```python
from build123d import *

# Parameters (mm, degrees)
F0_W     = 38.1
F0_H     = 19.05
F1_DEPTH = 3.175
F2_R     = 2.4828109925
F3_DEPTH = 3.176
F4_R     = 2.4828109925
F4_R_2   = 3.3973385268
F4_R_3   = 3.0356553695
F5_DEPTH = 0.254


with BuildPart() as f1:
    # F0 (on Top) → F1 (new body)
    with BuildSketch(Plane.XY):
        with Locations((-19.05, 9.525)):
            Rectangle(F0_W, F0_H)
    extrude(amount=F1_DEPTH)

    # F2 (on face) → F3 (cut, through all)
    with BuildSketch(Plane.XY.offset(3.175)):
        with BuildLine():
            ThreePointArc((-38.1, 9.525), (-35.2368913149, 16.0874822179), (-28.718682006, 19.05))
            Line((-28.718682006, 19.05), (-38.1, 19.05))
            Line((-38.1, 19.05), (-38.1, 9.525))
        make_face()
        with BuildLine():
            ThreePointArc((-28.718682006, 0), (-35.2368913149, 2.9625177821), (-38.1, 9.525))
            Line((-38.1, 9.525), (-38.1, 0))
            Line((-38.1, 0), (-28.718682006, 0))
        make_face()
        with Locations((-33.7038896978, 9.525)):
            Circle(F2_R)
    extrude(amount=-F3_DEPTH, mode=Mode.SUBTRACT)

    # F4 (on face) → F5 (cut)
    with BuildSketch(Plane.XY.offset(3.175)):
        with BuildLine():
            ThreePointArc((-28.718682006, 19.05), (-35.2368913149, 16.0874822179), (-38.1, 9.525))
            ThreePointArc((-38.1, 9.525), (-35.2368913149, 2.9625177821), (-28.718682006, 0))
            Line((-28.718682006, 0), (0, 0))
            Line((0, 0), (0, 19.05))
            Line((0, 19.05), (-28.718682006, 19.05))
        make_face()
        with Locations((-33.7038896978, 9.525)):
            Circle(F4_R, mode=Mode.SUBTRACT)
        with BuildLine():
            Line((-11.204509369, 9.7731091082), (-16.2556674331, 9.7731091082))
            Line((-16.2556674331, 9.7731091082), (-16.6581426853, 9.7731091082))
            ThreePointArc((-16.6581426853, 9.7731091082), (-24.1825202508, 10.7437230347), (-16.6363575836, 11.5271629766))
            Line((-16.6363575836, 11.5271629766), (-16.3941457868, 11.5271629766))
            Line((-16.3941457868, 11.5271629766), (-11.2256935624, 11.5271629766))
            ThreePointArc((-11.2256935624, 11.5271629766), (-3.4717256344, 10.7436549328), (-11.204509369, 9.7731091082))
        make_face(mode=Mode.SUBTRACT)
        with Locations((-7.3930802755, 10.6962956488)):
            Circle(F4_R_2)
        with BuildLine():
            add(Edge.make_bspline(
                [(-8.4561556578, 10.4526774958), (-8.4344821955, 10.5131812711), (-8.6159052615, 10.7046403164), (-8.9098232628, 10.8195179836), (-9.3586544368, 10.7286119848), (-9.574745931, 10.1187053668), (-9.2805338199, 9.538167958), (-8.8082365512, 9.5804816092), (-8.4556586549, 9.7438202932), (-8.396860102, 9.9863555926), (-8.6330082393, 10.0702183652), (-8.6519010809, 9.7333768373), (-9.0449295596, 9.7024764863), (-9.3441221135, 9.9584577723), (-9.3874655572, 10.524078357), (-8.9264365843, 10.6826697258), (-8.6368050913, 10.6049347389), (-8.6279642917, 10.3475627852), (-8.4719713543, 10.4085262966), (-8.4561556578, 10.4526774958)],
                knots=[0, 0, 0, 0, 0.0532483387, 0.113267174, 0.1785434515, 0.2577982567, 0.3354252403, 0.4027712128, 0.4668510982, 0.5116274353, 0.551372775, 0.6028604887, 0.6613225245, 0.7248177023, 0.7963036394, 0.8635278137, 0.9167089689, 0.9611432841, 1, 1, 1, 1], degree=3))
        make_face(mode=Mode.SUBTRACT)
        Polygon((-8.2311294973, 9.6275797114), (-8.2311294973, 10.7419975102), (-8.0918269232, 10.7741439715), (-8.0918269232, 9.7133042291), (-7.5239026919, 9.7133042291), (-7.5239026919, 9.6275797114), align=None, mode=Mode.SUBTRACT)
        with BuildLine():
            Line((-6.3773384318, 10.7741439715), (-6.3773384318, 10.6962956488))
            Line((-6.3773384318, 10.6962956488), (-6.3773384318, 9.9276155233))
            add(Edge.make_bspline(
                [(-6.3773384318, 9.9276155233), (-6.4090453416, 9.8087981466), (-6.480236508, 9.5420188336), (-7.1453746708, 9.5677405448), (-7.258420068, 9.8154754172), (-7.3095913976, 9.9276155233)],
                knots=[0, 0, 0, 0, 0.3053274615, 0.6855482984, 1, 1, 1, 1], degree=3))
            Line((-7.3095913976, 9.9276155233), (-7.2881602682, 10.7955755666))
            Line((-7.2881602682, 10.7955755666), (-7.1702892892, 10.7926651697))
            Line((-7.1702892892, 10.7926651697), (-7.1702892892, 9.9276155233))
            add(Edge.make_bspline(
                [(-7.1702892892, 9.9276155233), (-7.1284542088, 9.8465309767), (-7.0391238846, 9.6733913827), (-6.6129016247, 9.6843481722), (-6.5685332878, 9.8526930406), (-6.5487870015, 9.9276155233)],
                knots=[0, 0, 0, 0, 0.3283233699, 0.7010679257, 1, 1, 1, 1], degree=3))
            Line((-6.5487870015, 9.9276155233), (-6.5487870015, 10.7741439715))
            Line((-6.5487870015, 10.7741439715), (-6.3773384318, 10.7741439715))
        make_face(mode=Mode.SUBTRACT)
        with BuildLine():
            Line((-6.1201648787, 9.6168639138), (-6.1201648787, 10.6962956488))
            Line((-6.1201648787, 10.6962956488), (-6.1201648787, 10.8170062304))
            Line((-6.1201648787, 10.8170062304), (-5.577086471, 10.8170062304))
            add(Edge.make_bspline(
                [(-5.577086471, 10.8170062304), (-5.4622781191, 10.7638193061), (-5.2295052196, 10.6559832962), (-5.3677642589, 10.2445065322), (-5.5472345904, 10.2120818848), (-5.1332134299, 10.1753596302), (-5.270141809, 9.5907558618), (-5.4344035608, 9.6095224454), (-5.498662591, 9.6168639138)],
                knots=[0, 0, 0, 0, 0.1903840672, 0.3860019817, 0.4771127011, 0.6375520727, 0.8582107397, 1, 1, 1, 1], degree=3))
            Line((-5.498662591, 9.6168639138), (-6.1201648787, 9.6168639138))
        make_face(mode=Mode.SUBTRACT)
        with BuildLine():
            add(Edge.make_bspline(
                [(-8.5740266368, 12.2743221), (-8.5401050741, 12.3224331664), (-8.6783215627, 12.6387800293), (-9.184796294, 12.6548329665), (-9.4800471983, 12.4360053833), (-9.4419740945, 12.0798316165), (-9.1295950241, 11.9793082685), (-8.831367579, 11.9123580888), (-8.6427968335, 11.8238895712), (-8.7645291474, 11.5344085895), (-9.1140370755, 11.5542180365), (-9.3260330715, 11.6778761827), (-9.2954318773, 11.9042158216), (-9.5962395192, 11.8814661597), (-9.3559672194, 11.4482164997), (-8.9967184633, 11.3933195663), (-8.5558015163, 11.4768320471), (-8.5479985096, 11.8327800081), (-8.6951902579, 12.1024272986), (-9.0540613983, 12.0793081599), (-9.2629319892, 12.2276324709), (-9.3267172394, 12.4649328799), (-8.8420264537, 12.5231376903), (-8.7560312169, 12.2648192132), (-8.5972865041, 12.2413325519), (-8.5740266368, 12.2743221)],
                knots=[0, 0, 0, 0, 0.0453790473, 0.1028040475, 0.1504811039, 0.1945666876, 0.2403101145, 0.2875747753, 0.3209496051, 0.3604616335, 0.4077131796, 0.4470225316, 0.4812881885, 0.5136946038, 0.5632768855, 0.6145773714, 0.6660910242, 0.7111117469, 0.7544039284, 0.8020681877, 0.8434151076, 0.8768269994, 0.927247352, 0.9688837855, 1, 1, 1, 1], degree=3))
        make_face(mode=Mode.SUBTRACT)
        Polygon((-7.8090997019, 12.6045872655), (-7.6965680346, 12.5722642988), (-7.6278613442, 12.5489299599), (-7.3010693838, 11.5974660136), (-7.0933157741, 12.5945020797), (-6.9865938276, 12.5722642988), (-7.2293586095, 11.4072051531), (-7.363169454, 11.3742146641), (-7.6278613442, 12.4478163728), (-7.6953512616, 12.4672017992), (-7.9846717417, 11.4599391818), (-8.1668356434, 11.4599391818), (-8.4240091965, 12.5850727782), (-8.2739917561, 12.5850727782), (-8.2739917561, 12.5200599432), (-8.0941422122, 11.612218302), align=None, mode=Mode.SUBTRACT)
        Polygon((-6.5702181309, 12.5722642988), (-6.5702181309, 11.4599391818), (-6.7630982958, 11.4599391818), (-6.7630982958, 12.5850727782), align=None, mode=Mode.SUBTRACT)
        Polygon((-6.1533457451, 11.4599391818), (-6.2916139141, 11.4599391818), (-6.2916139141, 12.5722642988), (-6.0880184174, 12.5722642988), (-5.7344050147, 11.5992417559), (-5.3265071474, 12.5722642988), (-5.1879114471, 12.5850727782), (-5.1879114471, 11.4599391818), (-5.3265071474, 11.4888185353), (-5.3265071474, 12.4672017992), (-5.7022585534, 11.4599391818), (-5.7942554325, 11.4791086827), (-6.1533457451, 12.4672017992), align=None, mode=Mode.SUBTRACT)
        with Locations((-20.3638467938, 10.6962956488)):
            Circle(F4_R_3)
        Polygon((-22.3368285224, 10.0579196587), (-22.3368285224, 11.4144319668), (-22.9246504605, 11.4144319668), (-22.9246504605, 11.5953003988), (-21.7490065843, 11.5953003988), (-21.7490065843, 11.4144319668), (-22.165004164, 11.4144319668), (-22.165004164, 10.0579196587), align=None, mode=Mode.SUBTRACT)
        with BuildLine():
            add(Edge.make_bspline(
                [(-20.1857835054, 11.154637672), (-20.1383999259, 11.2274152197), (-20.3829405313, 11.5457368967), (-20.6342772805, 11.598445001), (-21.0338008973, 11.6033106802), (-21.3419507458, 11.4407849932), (-21.6690667935, 10.8714835234), (-21.4236479789, 10.2762233569), (-21.0513889722, 9.9385606622), (-20.5169842312, 10.0010364298), (-20.3022849329, 10.2346080768), (-20.0935529686, 10.5076427388), (-20.4542795834, 10.6178192925), (-20.4380739541, 10.1568095491), (-21.0016529566, 10.1732881394), (-21.3412121983, 10.4615670014), (-21.3344036941, 10.8906002083), (-21.2656345796, 11.2749928339), (-20.8158403075, 11.5352908662), (-20.428962716, 11.3142068841), (-20.4926924052, 11.1040132427), (-20.2235079909, 11.0966957528), (-20.1857835054, 11.154637672)],
                knots=[0, 0, 0, 0, 0.0513054787, 0.0956974598, 0.1461415157, 0.1942748513, 0.2581448225, 0.3224312905, 0.3794034791, 0.4364585944, 0.4844359856, 0.5259974197, 0.5628941445, 0.6093371792, 0.6648394213, 0.7183478226, 0.7706084866, 0.8213935407, 0.8774060244, 0.9271153733, 0.9591530905, 1, 1, 1, 1], degree=3))
        make_face(mode=Mode.SUBTRACT)
        Polygon((-19.6997895837, 10.0419670343), (-19.929997623, 10.0579196587), (-19.929997623, 11.5766851231), (-19.7125785053, 11.5766851231), (-18.8940633088, 10.4000680149), (-18.8940633088, 11.5766851231), (-18.6894331127, 11.5766851231), (-18.6894331127, 10.0419670343), (-18.9835876226, 10.0419670343), (-19.6997895837, 11.1674275249), align=None, mode=Mode.SUBTRACT)
        with BuildLine():
            Line((-17.589552328, 11.5894749761), (-17.589552328, 11.487159878))
            Line((-17.589552328, 11.487159878), (-17.589552328, 10.3744892403))
            add(Edge.make_bspline(
                [(-17.806969583, 10.3744892403), (-17.8318558411, 10.3003918473), (-17.8864489425, 10.1378440474), (-18.3385288849, 10.2040992572), (-18.1812855735, 10.5182028777), (-18.5826669281, 10.5557536384), (-18.4155770482, 10.0550453731), (-18.0308547555, 9.9537773156), (-17.6795258923, 10.070041505), (-17.619054133, 10.2746626102), (-17.589552328, 10.3744892403)],
                knots=[0, 0, 0, 0, 0.1092025201, 0.2395580825, 0.3484827985, 0.4538953578, 0.5953349525, 0.7397365792, 0.8730276614, 1, 1, 1, 1], degree=3))
            Line((-17.806969583, 10.3744892403), (-17.806969583, 11.5894749761))
            Line((-17.806969583, 11.5894749761), (-17.589552328, 11.5894749761))
        make_face(mode=Mode.SUBTRACT)
        with BuildLine():
            Line((-5.9947180562, 10.1604396477), (-5.9594316408, 9.7347348928))
            Line((-5.9594316408, 9.7347348928), (-5.5234750036, 9.686926615))
            add(Edge.make_bspline(
                [(-5.577086471, 10.1604396477), (-5.4947674906, 10.1405781416), (-5.3197424976, 10.098348999), (-5.3898233796, 9.7815677736), (-5.4865108779, 9.7080351973), (-5.5234750036, 9.686926615)],
                knots=[0, 0, 0, 0, 0.3268123342, 0.6948619404, 0.9017848331, 0.9017848331, 0.9017848331, 0.9017848331], degree=3))
            Line((-5.577086471, 10.1604396477), (-5.9947180562, 10.1604396477))
        make_face()
        with BuildLine():
            Line((-5.4772314616, 10.6562729925), (-5.9701469727, 10.6562729925))
            Line((-5.9701469727, 10.6562729925), (-5.9701469727, 10.2705126628))
            Line((-5.9701469727, 10.2705126628), (-5.577086471, 10.2705126628))
            add(Edge.make_bspline(
                [(-5.4772314616, 10.6562729925), (-5.4643446002, 10.6041130472), (-5.4353366378, 10.486702477), (-5.5264502908, 10.3477404531), (-5.577086471, 10.2705126628)],
                knots=[0, 0, 0, 0, 0.4442525507, 1, 1, 1, 1], degree=3))
        make_face()
    extrude(amount=-F5_DEPTH, mode=Mode.SUBTRACT)


solid = f1.part
```
Check sheet for the modelled part. Datum: model origin and axes. Units: mm. A direction names the side the tool comes from. Round coordinates to 2 decimals unless told otherwise and drop trailing zeros. Write each loop counter-clockwise with the first axis right and the second up, starting at its lowest first coordinate (ties: lowest second). Pieces come first, ordered by that corner, then holes. Notation, with made-up numbers: (-28, 87) -> (-11, 87) arc R23 cw to (-11, 104) -> close; hole circle Ø9 at (32, 19.5). An arc over 180 degrees is marked (long way). Put each result on its own line as item: value.
(1) Sectioned sample at A-A (z = 0.65). Enter the section's corners in (x, y) (3 decimals).
Values found:
outline: (-38.1, 9.525) arc R9.992 ccw to (-28.719, 0) -> (0, 0) -> (0, 19.05) -> (-28.719, 19.05) arc R9.992 ccw to start; hole circle Ø4.966 at (-33.704, 9.525)
(2) Material ranges on line 1 (Z direction, x = -15, y = 1.75); line 2 (X direction, y = 8.75, z = 2.5); line 3 (X direction, y = 3.5, z = 0.45), recorded low to high.
Values found:
line 1: z = 0 to 2.92
line 2: x = -38.03 to -36.06, -31.35 to 0
line 3: x = -35.73 to 0
(3) Tool access check on faces 1 (the face through (-15, 19.05, 1)), 2 (the face through (-19, 5, 2.921)). Record the directions out of +Z, -Z, +X, -X, +Y, -Y that give a thin tool (end or side, any length) a straight path to the whole face; none if there is none.
Values found:
face 1: +Z, -Z, +X, -X, +Y
face 2: +Z
(4) Sectioned sample at B-B (x = -13). Enter the section's corners in (y, z) (3 decimals), plus the area to 3 significant figures.
Values found:
outline: (0, 0) -> (19.05, 0) -> (19.05, 2.921) -> (11.527, 2.921) -> (11.527, 3.175) -> (9.773, 3.175) -> (9.773, 2.921) -> (0, 2.921) -> close
area: 56.1 mm^2
(5) Sectioned sample at D-D (y = 3.5). Enter the section's corners in (x, z).
Values found:
outline: (-35.73, 0) -> (0, 0) -> (0, 2.92) -> (-35.73, 2.92) -> close
(6) Go/stop test with a flat-tipped pin: pin 1 Ø1 at (x, y) = (-20, 4) entering from +Z. Record where the tip stops, or that it passes through.
Values found:
pin 1: stops at z = 2.92
(7) Sectioned sample at C-C (y = 13). Enter the section's corners in (x, z) (3 decimals).
Values found:
outline: (-37.307, 0) -> (0, 0) -> (0, 2.921) -> (-4.219, 2.921) -> (-4.219, 3.175) -> (-4.896, 3.175) -> (-4.896, 2.921) -> (-9.89, 2.921) -> (-9.89, 3.175) -> (-10.567, 3.175) -> (-10.567, 2.921) -> (-17.318, 2.921) -> (-17.318, 3.175) -> (-18.387, 3.175) -> (-18.387, 2.921) -> (-22.341, 2.921) -> (-22.341, 3.175) -> (-23.41, 3.175) -> (-23.41, 2.921) -> (-37.307, 2.921) -> close
(8) Mould release check, pull along Y, two halves, no side actions. Record for faces 3 (the face through (-15, 11, 3.175)), 4 (the face through (-35.31, 16.01, 1.48)), 5 (the face through (-36.184, 9.634, 1.481)): released by +Y, released by -Y, zero draft, split by the parting line, or undercut.
Values found:
face 3: zero draft
face 4: released by +Y
face 5: undercut
